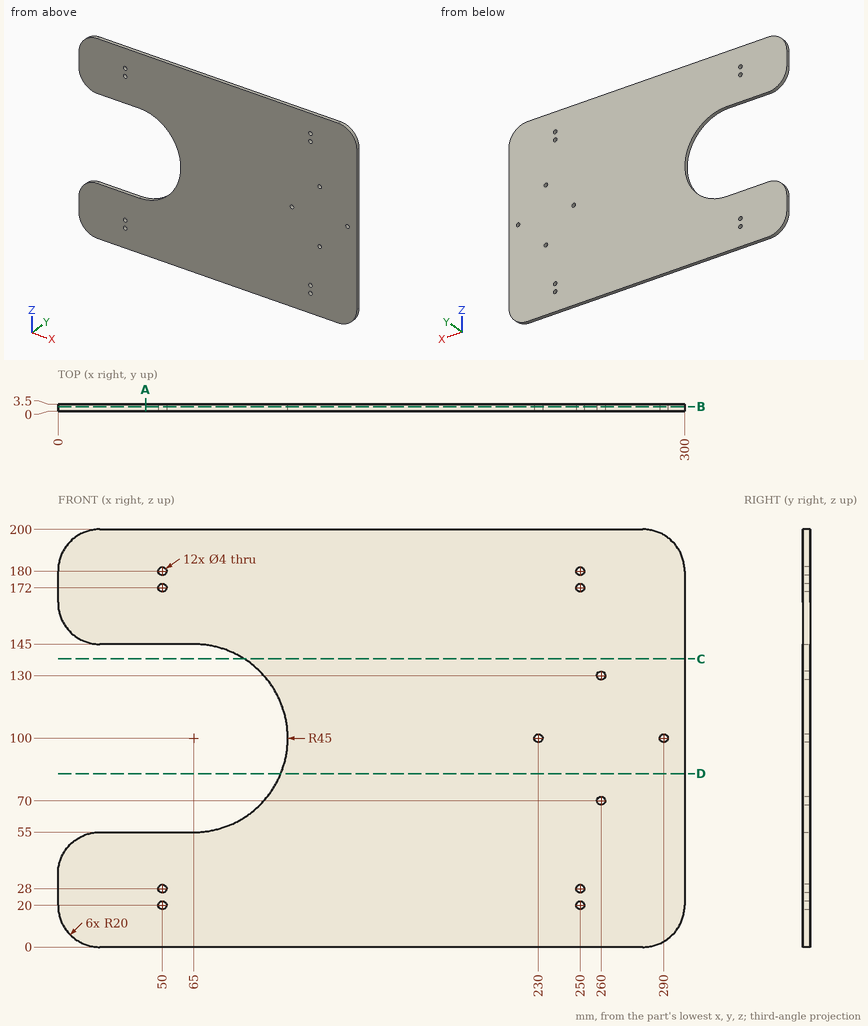
For this review, use the dimensioned drawing (mm, ordinates from the lowest corner) and the shaded views. Round coordinates to 2 decimals unless told otherwise and drop trailing zeros. Loops run counter-clockwise (first coordinate to the right, second up) from the corner with the lowest first, then second, coordinate; pieces in that order, holes last. Notation, with made-up numbers: M 45,8 L 73,8 A26 ccw 73,46 Z; hole C 77.5,53.5 d4. An arc over 180 degrees is marked long. Answer as CSV lines item,"result".
1. To check wall thickness, follow L1, parallel to X at y = 1.4, z = 28; L2, parallel to Z at x = 250, y = 2.65; L3, parallel to Z at x = 260, y = 1.2. State the ranges of each line that lie inside material, in increasing order. Write a range as [from, to].
Outcome:
L1,"x = [0, 48], [52, 248], [252, 300]"
L2,"z = [0, 18], [22, 26], [30, 170], [174, 178], [182, 200]"
L3,"z = [0, 68], [72, 128], [132, 200]"
2. We need section B-B (y = 2.2). Count the separate pieces of the cut face and the enclosed holes in it, plus the area to 3 significant figures.
Outcome:
separate pieces,"1"
enclosed holes,"12"
area,"50,300 mm2"
3. We need section A-A (x = 42). Give the boundary of the cut face in (y, z), plus the area to 3 significant figures.
Outcome:
outline,"M 0,0 L 3.5,0 L 3.5,55 L 0,55 Z; M 0,145 L 3.5,145 L 3.5,200 L 0,200 Z"
area,"385 mm2"
4. Insertion check: pin 1 Ø1.5 at (y, z) = (2.5, 80.5) entering from -X; pin 2 Ø3.5 at (x, z) = (290, 100) entering from +Y. Each pin has a flat end and moves straight along its axis. Give the tip position at first contact, or say it passes through.
Outcome:
pin 1,"stops at x = 105.19"
pin 2,"passes through"
5. We need section C-C (z = 138). Give the boundary of the cut face in (x, y).
Outcome:
outline,"M 89.1,0 L 300,0 L 300,3.5 L 89.1,3.5 Z"
6. We need section D-D (z = 83). Give the boundary of the cut face in (x, y).
Outcome:
outline,"M 106.67,0 L 300,0 L 300,3.5 L 106.67,3.5 Z"
